from build123d import *

# Parameters (mm, degrees)
SKETCH1_W           = 80
SKETCH1_H           = 50
BOSS_EXTRUDE1_DEPTH = 5
SKETCH4_R           = 11
BOSS_EXTRUDE2_DEPTH = 10
SKETCH5_R           = 11
SKETCH5_R_2         = 6
BOSS_EXTRUDE3_DEPTH = 5
BOSS_EXTRUDE4_DEPTH = 5
FILLET2_R           = 7
SKETCH7_R           = 2
CUT_EXTRUDE1_DEPTH  = 5
FILLET3_R           = 5


with BuildPart() as part:
    # Sketch1 → Boss-Extrude1 (new body)
    with BuildSketch(Plane(origin=(0, 0, 0), x_dir=(1, 0, 0), z_dir=(0, 1, 0))):
        Rectangle(SKETCH1_W, SKETCH1_H)
    extrude(amount=BOSS_EXTRUDE1_DEPTH)

    # Sketch4 → Boss-Extrude2 (add)
    with BuildSketch(Plane.XY.offset(25)):
        with BuildLine():
            Line((-20, 25), (-20, 5))
            Line((-20, 5), (20, 5))
            Line((20, 5), (20, 25))
            ThreePointArc((20, 25), (0, 45), (-20, 25))
        make_face()
        with Locations((0, 25)):
            Circle(SKETCH4_R, mode=Mode.SUBTRACT)
    extrude(amount=-BOSS_EXTRUDE2_DEPTH)

    # Sketch5 → Boss-Extrude3 (add)
    with BuildSketch(Plane.XY.offset(25)):
        with Locations((0, 25)):
            Circle(SKETCH5_R)
        with Locations((0, 25)):
            Circle(SKETCH5_R_2, mode=Mode.SUBTRACT)
    extrude(amount=-BOSS_EXTRUDE3_DEPTH)

    # Sketch6 → Boss-Extrude4 (add)
    with BuildSketch(Plane.ZY.offset(20)):
        Polygon((15, 25), (-19.641016151, 5), (15, 5), align=None)
    boss_extrude4 = extrude(amount=-BOSS_EXTRUDE4_DEPTH)

    # Mirror1: Boss-Extrude4 across plane
    add(boss_extrude4.mirror(Plane(origin=(0, 0, 0), x_dir=(0, 0, 1), z_dir=(1, 0, 0))))

    # Fillet2
    fillet2_edges = [part.edges().sort_by_distance(p)[0] for p in [
        (0, 5, 15),
        (-17.5, 25, 15),
        (-17.5, 5, -19.641016151),
        (17.5, 25, 15),
        (17.5, 5, -19.641016151),
    ]]
    fillet(fillet2_edges, radius=FILLET2_R)

    # Sketch7 → Cut-Extrude1 (cut)
    with BuildSketch(Plane.XZ):
        with Locations(Location((-32.5, 20, 0), (0, 0, 270))):
            Circle(SKETCH7_R)
        with Locations(Location((-32.5, -20, 0), (0, 0, 270))):
            Circle(SKETCH7_R)
        with Locations(Location((32.5, -20, 0), (0, 0, 270))):
            Circle(SKETCH7_R)
        with Locations(Location((32.5, 20, 0), (0, 0, 270))):
            Circle(SKETCH7_R)
    extrude(amount=-CUT_EXTRUDE1_DEPTH, mode=Mode.SUBTRACT)

    # Fillet3
    fillet3_edges = [part.edges().sort_by_distance(p)[0] for p in [
        (40, 2.5, 25),
        (-40, 2.5, 25),
        (-40, 2.5, -25),
        (40, 2.5, -25),
    ]]
    fillet(fillet3_edges, radius=FILLET3_R)


solid = part.part
The model under review builds one solid part; all positions refer to its coordinate system, in mm. A direction names the side the tool comes from. Give positions to 0.01 mm unless a question says otherwise; leave off trailing zeros. Loops run counter-clockwise (first coordinate to the right, second up) from the corner with the lowest first, then second, coordinate; pieces in that order, holes last. Notation, with made-up numbers: (-38, 3) -> (7, 3) arc R17 ccw to (7, 27) -> close; hole circle Ø5 at (33.5, 13). An arc over 180 degrees is marked (long way). Put each result on its own line as item: value. Start each with the question number.
1. We need section C-C on x = 0. State the section outline as (y, z) points.
2. We need section D-D on z = -7. State the section outline as (x, y) points.
3. Clearance check with flat-ended pins moving along their axes: P1, Ø15.5, axis at x = 0, y = 25, coming from the +Z side; P2, Ø10, axis at y = 13.5, z = 3.5, coming from the +X side; P3, Ø1.5, axis at x = 30.5, z = 13.5, coming from the +Y side; P4, Ø6, axis at y = 16.5, z = 9, coming from the -X side. State where each tip first meets the part, or that it passes through.
4. We need section A-A on x = -32.5. State the section outline as (y, z) points.
5. Mouldability with a two-part tool opening along Y and no side actions: class faces 4 (the face through (17.54, 14.58, -3.05)), 5 (the face through (5, 20, 20)), 6 (the face through (-20, 13, 12)) as released by +Y, released by -Y, zero draft, split by the parting line, or undercut.
6. Wall thickness on probe 1 along X at (y, z) = (2.5, -20); probe 2 along Y at (x, z) = (0, 23.05); probe 3 along Z at (x, y) = (-32, 2): over which ranges is each line inside the solid? List them lowest first.
7. For faces 1 (the face through (-2.38, 14.26, 17.54)), 2 (the face through (-15, 12, 5)), 3 (the face through (17.46, 25.5, 14.04)), list the 3-axis set-ups (+Z, -Z, +X, -X, +Y, -Y) from which the entire face can be reached by the end or side of a thin tool; tool diameter is ignored.
8. We need section B-B on y = 28. State the section outline as (x, z) points, then the cut area to 3 significant figures.
Determined:
1. outline: (0, -25) -> (5, -25) -> (5, 8) arc R7 cw to (12, 15) -> (14, 15) -> (14, 20) -> (19, 20) -> (19, 25) -> (0, 25) -> close; (31, 20) -> (36, 20) -> (36, 15) -> (45, 15) -> (45, 25) -> (31, 25) -> close
2. outline: (-40, 0) -> (40, 0) -> (40, 5) -> (20, 5) -> (20, 12.3) -> (15, 12.3) -> (15, 5) -> (-15, 5) -> (-15, 12.3) -> (-20, 12.3) -> (-20, 5) -> (-40, 5) -> close
3. P1: z = 25
3. P2: x = 20
3. P3: y = 5
3. P4: x = -20
4. outline: (0, -25) -> (5, -25) -> (5, -22) -> (0, -22) -> close; (0, -18) -> (5, -18) -> (5, 18) -> (0, 18) -> close; (0, 22) -> (5, 22) -> (5, 25) -> (0, 25) -> close
5. face 4: released by +Y
5. face 5: undercut
5. face 6: zero draft
6. probe 1: -40 to -34.5, -30.5 to 30.5, 34.5 to 40
6. probe 2: 0 to 19, 31 to 45
6. probe 3: -25 to -21.94, -18.06 to 18.06, 21.94 to 25
7. face 1: -Z
7. face 2: -Z, +Y
7. face 3: -Z, +X, -X, +Y
8. outline: (-19.77, 14.92) -> (-15, 14.92) -> (-15, 15) -> (-10.58, 15) -> (-10.58, 20) -> (-5.2, 20) -> (-5.2, 25) -> (-19.77, 25) -> close; (5.2, 20) -> (10.58, 20) -> (10.58, 15) -> (15, 15) -> (15, 14.92) -> (19.77, 14.92) -> (19.77, 25) -> (5.2, 25) -> close
8. area: 238 mm^2
